Part print with two shaded views. Sizes in mm from the minimum x, y, z corner. A direction names the side the tool comes from. Round coordinates to 2 decimals unless told otherwise and drop trailing zeros. Loops run counter-clockwise (first coordinate to the right, second up) from the corner with the lowest first, then second, coordinate; pieces in that order, holes last. Notation, with made-up numbers: M 1,22 L 46,22 A6 ccw 46,28 Z; hole C -18.5,75 d4. An arc over 180 degrees is marked long. Answer as CSV lines item,"result". Start each with the question number.
Item 1: Band-saw the part on D-D (z = 128). Give the cut face in (x, y) (1 decimal).
Item 2: Which spindle directions (+Z, -Z, +X, -X, +Y, -Y) get a long thin tool onto all of the face, cutting with end or side? Do the marked faces 4 and 5. Say none if no direction does.
Item 3: Mould opens along Z. For the marked faces 1, 2 and 3 say: pulls with the +Z half, pulls with the -Z half, needs draft (parallel to the pull), parting line crosses it, or undercut.
Item 4: Band-saw the part on C-C (y = 8.25). Give the cut face in (x, z) (1 decimal).
Item 5: Band-saw the part on A-A (x = 44). Give the cut face in (y, z) (1 decimal).
Item 6: Drop flat-ended pins along their axis: pin 1 Ø3 at (y, z) = (5, 57.5) entering from -X; pin 2 Ø6 at (x, y) = (91, 13.5) entering from -Z; pin 3 Ø8 at (y, z) = (13, 125) entering from +X (1 decimal); pin 4 Ø8 at (x, z) = (47.5, 127) entering from -Y. Give the stop position or say it passes through.
Item 7: Wall check: line 1 (X direction, y = 3.5, z = 51); line 2 (X direction, y = 18.5, z = 124.5) (1 decimal); line 3 (X direction, y = 22.75, z = 31) (1 decimal). Give the ranges that are in metal, low to high.
Item 8: Band-saw the part on B-B (z = 71). Give the cut face in (x, y) (1 decimal), and give its area (3 significant figures).
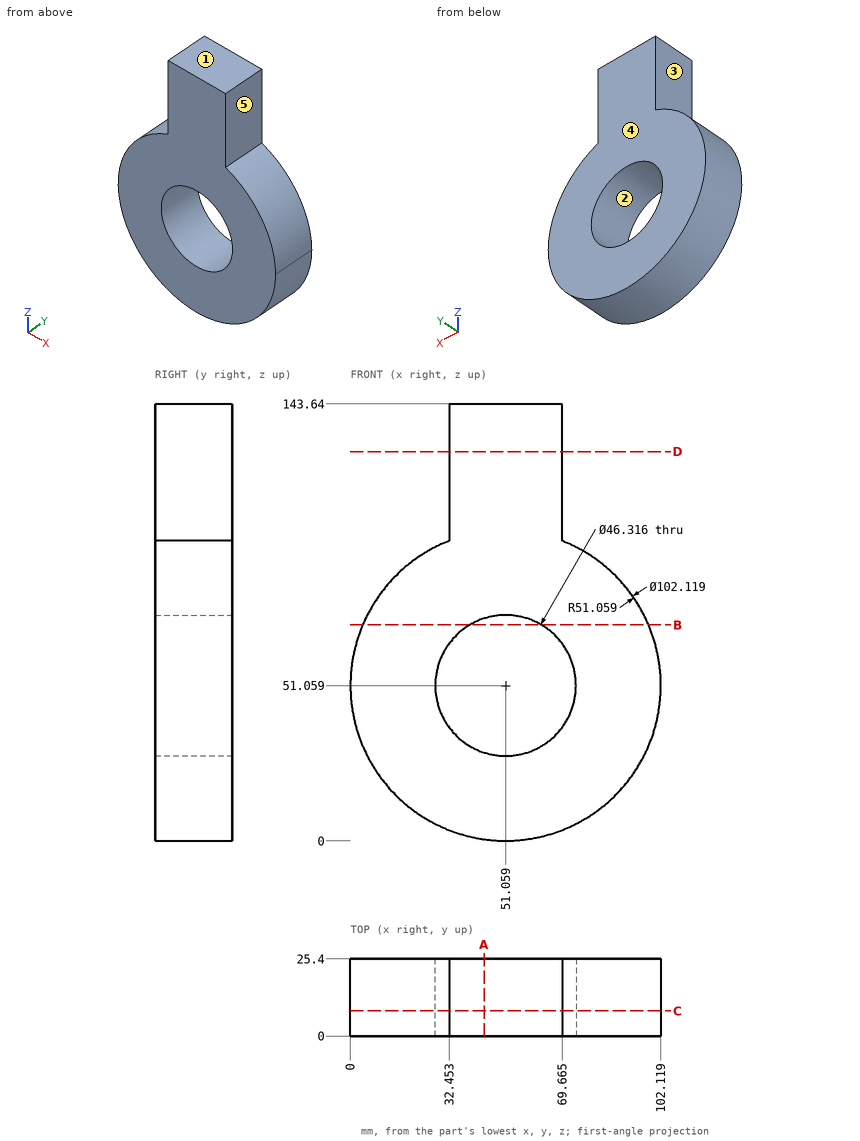
Answer block:
1,outline,"M 32.5,0 L 69.7,0 L 69.7,25.4 L 32.5,25.4 Z"
2,face 4,"+Z, -Z, +X, -X, +Y"
2,face 5,"+Z, +X, +Y, -Y"
3,face 1,"pulls with the +Z half"
3,face 2,"undercut"
3,face 3,"needs draft"
4,outline,"M 32.5,98.6 A51.1 ccw long 69.7,98.6 L 69.7,143.6 L 32.5,143.6 Z; hole C 51.1,51.1 d46.3"
5,outline,"M 0,0.5 L 25.4,0.5 L 25.4,29 L 0,29 Z; M 0,73.1 L 25.4,73.1 L 25.4,143.6 L 0,143.6 Z"
6,pin 1,"stops at x = 0.24"
6,pin 2,"stops at z = 15.81"
6,pin 3,"stops at x = 69.7"
6,pin 4,"stops at y = 0"
7,line 1,"x = 0 to 27.9, 74.22 to 102.12"
7,line 2,"x = 32.5 to 69.7"
7,line 3,"x = 4.1 to 39.5, 62.6 to 98"
8,outline,"M 4.1,0 L 39.3,0 L 39.3,25.4 L 4.1,25.4 Z; M 62.8,0 L 98.1,0 L 98.1,25.4 L 62.8,25.4 Z"
8,area,"1,790 mm^2"
